Input: dimensioned drawing with shaded views. Units: mm. Origin: part minimum x, y, z. A direction names the side the tool comes from. Give positions to 0.01 mm unless a question says otherwise; leave off trailing zeros. Order: outer loops, then holes, each group sorted by start corner. A loop starts at its lowest first (then second) coordinate and runs counter-clockwise, first axis right, second up. Notation, with made-up numbers: (-31, 23.25) - (-1, 23.25) arc R18 ccw to (-1, 28.25) - close; hole circle Ø1 at (5.25, 62.25). An arc over 180 degrees is marked (long way). Answer as CSV lines item,"result".
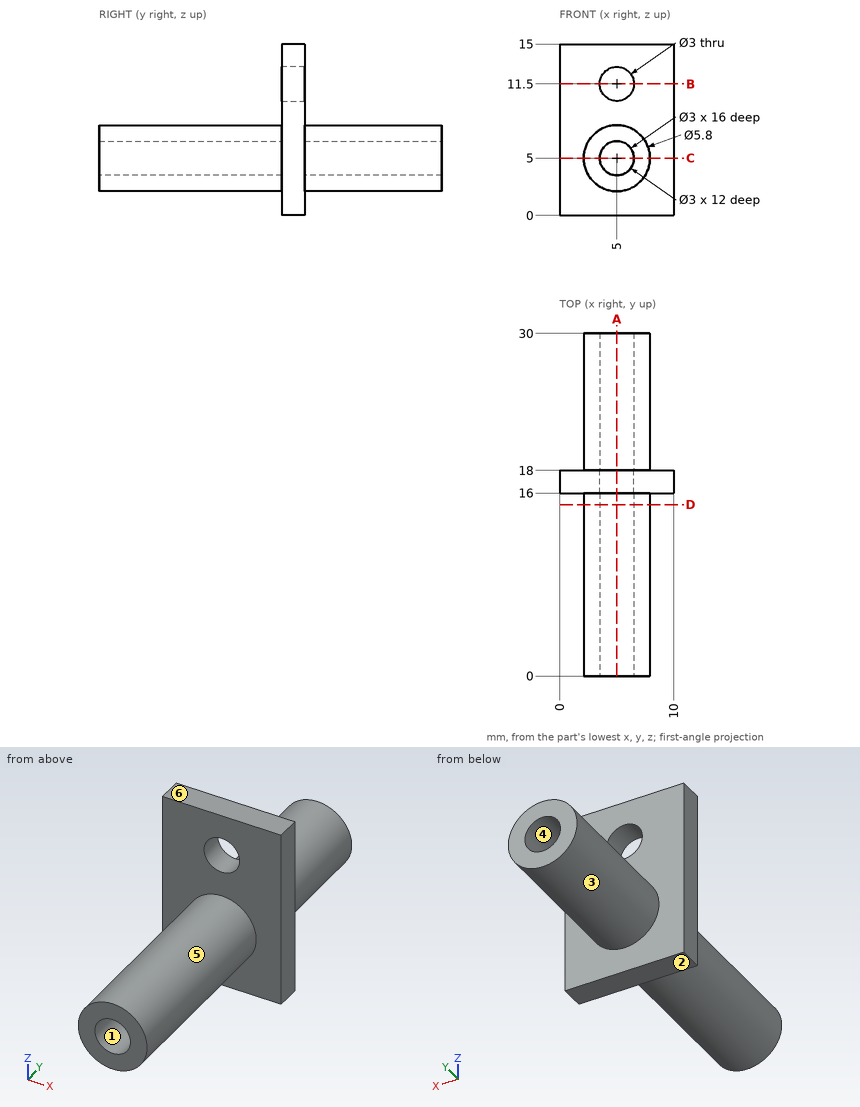
(1) Cut plane D-D (y = 15). Return loops of the section in (x, z).
Completed:
outline,"circle Ø5.8 at (5, 5); hole circle Ø3 at (5, 5)"
(2) Cut plane A-A (x = 5). Return loops of the section in (y, z).
Completed:
outline,"(0, 2.1) - (16, 2.1) - (16, 0) - (18, 0) - (18, 2.1) - (30, 2.1) - (30, 3.5) - (18, 3.5) - (18, 6.5) - (30, 6.5) - (30, 7.9) - (18, 7.9) - (18, 10) - (16, 10) - (16, 7.9) - (0, 7.9) - (0, 6.5) - (16, 6.5) - (16, 3.5) - (0, 3.5) - close; (16, 13) - (18, 13) - (18, 15) - (16, 15) - close"
(3) Mould query, pull axis Z, two halves, no side actions, for the marked faces 1, 2 and 3. Classes: released by +Z, released by -Z, zero draft, split by the parting line, or undercut.
Completed:
face 1,"undercut"
face 2,"released by -Z"
face 3,"split by the parting line"
(4) Access query for the marked faces 4, 5 and 6. Directions: +Z, -Z, +X, -X, +Y, -Y. A direction counts if a zero-diameter tool reaches every point of the face in a straight line with its end or side. Return the directions, or none.
Completed:
face 4,"+Y"
face 5,"-Y"
face 6,"+Z, +X, -X, +Y, -Y"
(5) Cut plane C-C (z = 5). Return loops of the section in (x, y), then the cut area to 3 significant figures.
Completed:
outline,"(0, 16) - (2.1, 16) - (2.1, 0) - (3.5, 0) - (3.5, 16) - (6.5, 16) - (6.5, 0) - (7.9, 0) - (7.9, 16) - (10, 16) - (10, 18) - (7.9, 18) - (7.9, 30) - (6.5, 30) - (6.5, 18) - (3.5, 18) - (3.5, 30) - (2.1, 30) - (2.1, 18) - (0, 18) - close"
area,"98.4 mm²"
(6) Cut plane B-B (z = 11.5). Return loops of the section in (x, y), then the cut area to 3 significant figures.
Completed:
outline,"(0, 16) - (3.5, 16) - (3.5, 18) - (0, 18) - close; (6.5, 16) - (10, 16) - (10, 18) - (6.5, 18) - close"
area,"14.0 mm²"
(7) Contact query for flat-ended pins moving along their axis: pin 1 (1.8 mm diameter, centred on x = 5, z = 5, fed in from -Y); pin 2 (1.5 mm diameter, centred on y = 3.5, z = 7.5, fed in from +X); pin 3 (6 mm diameter, centred on x = 5.5, z = 12.5, fed in from +Y); pin 4 (1 mm diameter, centred on x = 5.5, z = 11.5, fed in from -Y). Output: stop coordinate, or through.
Completed:
pin 1,"y = 16"
pin 2,"x = 7.31"
pin 3,"y = 18"
pin 4,"through"
(8) Ray query, line 1 (X direction, y = 3.5, z = 5); line 2 (Y direction, x = 1.5, z = 12). Return the intervals inside material, ascending. Write a range as from..to.
Completed:
line 1,"2.1..3.5, 6.5..7.9"
line 2,"16..18"
